Here's how the part is built. I have some questions about the finished solid (model axes, mm). A direction names the side the tool comes from. Round coordinates to 2 decimals unless told otherwise and drop trailing zeros. Write each loop counter-clockwise with the first axis right and the second up, starting at its lowest first coordinate (ties: lowest second). Pieces come first, ordered by that corner, then holes. Notation, with made-up numbers: (41.5, -32.5) - (81.5, -32.5) arc R22 ccw to (81.5, -9.5) - close; hole circle Ø4 at (30, 73). An arc over 180 degrees is marked (long way). One line per question, with ' | ' between items. Start each with the question number.
(1) Will these pins go through, and if not, where does the flat tip stop? pin 1 (4 mm diameter, centred on x = -30, y = 10.5, fed in from +Z); pin 2 (5 mm diameter, centred on y = 13.5, z = -8, fed in from -X); pin 3 (1.5 mm diameter, centred on y = 0.5, z = 3.5, fed in from -X).
(2) For faces 1 (the flat face through (-41, 7.874, -4)), 2 (the cylindrical face through (7.7, 9.4, 10.1)), 3 (the cylindrical face through (-53.7, 48.96, -10.85)), which set-ups out of +Z, -Z, +X, -X, +Y, -Y let a thin tool reach every point of the face, with its end or its side?
(3) Imagine slicing it at A-A (z = 5). Write out the boundary of the cut face in (x, y).
(4) Imagine slicing it at B-B (x = -62.5). Write out the boundary of the cut face in (y, z).
(5) Imagine slicing it at C-C (y = 30.5). Write out the boundary of the cut face in (x, z).
(6) Thinking about a two-plate mould opening in Y: for faces 4 (the flat face through (-54, 26, -15.748)), 5 (the cylindrical face through (-38.323, 10.917, -10.854)), 6 (the cylindrical face through (-44.93, 49.75, -10.85)), which applies, pulls with the +Y half, pulls with the -Y half, needs draft (parallel to the pull), parting line crosses it, or undercut?
(7) Imagine slicing it at D-D (x = -43). Write out the boundary of the cut face in (y, z), plus the area to 3 significant figures.
(8) If I drill on L1, parallel to Y at x = -73.5, z = -11; L2, parallel to Z at x = -84.5, y = 44.5; L3, parallel to Y at x = -86, z = -8.5, over which ranges is the centre line in solid material (lowest first)?
from build123d import *

# Parameters (mm, degrees)
SALIENTE_EXTRUIR1_DEPTH      = 7.874
SALIENTE_EXTRUIR2_DEPTH      = 12.7
SALIENTE_EXTRUIR2_DEPTH_BACK = 12.7
CROQUIS4_R                   = 12.7
SALIENTE_EXTRUIR4_DEPTH      = 9.652
CORTAR_EXTRUIR1_DEPTH        = 9.652
CROQUIS10_R                  = 12.7
SALIENTE_EXTRUIR5_DEPTH      = 3.048


with BuildPart() as part:
    # Croquis2 → Saliente-Extruir1 (new body)
    with BuildSketch(Plane(origin=(0, 0, 0), x_dir=(1, 0, 0), z_dir=(0, 1, 0))):
        with BuildLine():
            Line((0, 15.748), (-88.9, 15.748))
            Line((-88.9, 15.748), (-88.9, -3.556))
            Line((-88.9, -3.556), (-24.886815787, -3.556))
            ThreePointArc((-24.886815787, -3.556), (-17.958619485, -5.161878518), (-12.443407893, -9.652))
            ThreePointArc((-12.443407893, -9.652), (14.142121482, -6.928196302), (0, 15.748))
        make_face()
    extrude(amount=SALIENTE_EXTRUIR1_DEPTH)

    # Croquis4 → Saliente-Extruir2 (add, two sides: drawn at the far end of the back side and taken through both)
    with BuildSketch(Plane.XY.offset(-6.096).offset(-SALIENTE_EXTRUIR2_DEPTH_BACK)):
        with Locations((-88.9, 3.937)):
            Circle(CROQUIS4_R)
    extrude(amount=SALIENTE_EXTRUIR2_DEPTH + SALIENTE_EXTRUIR2_DEPTH_BACK)

    # Croquis8 → Saliente-Extruir4 (add)
    with BuildSketch(Plane.XY.offset(-6.096)):
        with BuildLine():
            Line((-51.003957581, 7.874), (-25.522164513, 7.874))
            ThreePointArc((-25.522164513, 7.874), (-45.412930083, 50.209289224), (-88.9, 67.437))
            ThreePointArc((-88.9, 67.437), (-101.6, 54.737), (-88.9, 42.037))
            ThreePointArc((-88.9, 42.037), (-63.389117028, 32.235495543), (-51.003957581, 7.874))
        make_face()
    extrude(amount=-SALIENTE_EXTRUIR4_DEPTH)

    # Croquis9 → Cortar-Extruir1 (cut)
    with BuildSketch(Plane.XY.offset(-6.096)):
        with BuildLine():
            ThreePointArc((-88.9, 61.087), (-95.25, 54.737), (-88.9, 48.387))
            ThreePointArc((-88.9, 48.387), (-61.840554481, 39.201555976), (-45.964597021, 15.441506555))
            ThreePointArc((-45.964597021, 15.441506555), (-38.187467088, 10.951378494), (-33.697339028, 18.728508428))
            ThreePointArc((-33.697339028, 18.728508428), (-54.109284332, 49.277143398), (-88.9, 61.087))
        make_face()
    extrude(amount=-CORTAR_EXTRUIR1_DEPTH, mode=Mode.SUBTRACT)

    # Croquis10 → Saliente-Extruir5 (add)
    with BuildSketch(Plane(origin=(0, 7.874, 0), x_dir=(1, 0, 0), z_dir=(0, 1, 0))):
        with Locations(Location((0, 0, 0), (0, 0, 90))):
            Circle(CROQUIS10_R)
    extrude(amount=SALIENTE_EXTRUIR5_DEPTH)


solid = part.part
Check sheet entries:
1) pin 1: z = -6.1 | pin 2: x = -99.45 | pin 3: x = -101.31
2) face 1: none | face 2: +Y | face 3: +Z, -Z
3) outline: circle Ø25.4 at (-88.9, 3.94); (-18.3, 0) - (14.93, 0) - (14.93, 7.87) - (11.67, 7.87) - (11.67, 10.92) - (-11.67, 10.92) - (-11.67, 7.87) - (-18.3, 7.87) - close
4) outline: (0, -15.75) - (7.87, -15.75) - (7.87, 3.56) - (0, 3.56) - close; (31.41, -15.75) - (39.7, -15.75) - (39.7, -6.1) - (31.41, -6.1) - close; (54.62, -15.75) - (61.69, -15.75) - (61.69, -6.1) - (54.62, -6.1) - close
5) outline: (-61.59, -15.75) - (-53.26, -15.75) - (-53.26, -6.1) - (-61.59, -6.1) - close; (-38.3, -15.75) - (-31.22, -15.75) - (-31.22, -6.1) - (-38.3, -6.1) - close
6) face 4: needs draft | face 5: undercut | face 6: pulls with the +Y half
7) outline: (0, -15.75) - (11.58, -15.75) - (11.58, -6.1) - (7.87, -6.1) - (7.87, 3.56) - (0, 3.56) - close; (37.99, -15.75) - (47.82, -15.75) - (47.82, -6.1) - (37.99, -6.1) - close | area: 283 mm^2
8) L1: 0 to 7.87, 38.79 to 45.63, 58.97 to 65.54 | L2: -15.75 to -6.1 | L3: -8.43 to 16.3, 41.93 to 48.29, 61.01 to 67.37
